```python
from build123d import *

# Parameters (mm, degrees)
SKETCH_1_W          = 20
SKETCH_1_H          = 20
SKETCH_1_R          = 1
EXTRUDE_1_DEPTH     = 28
EXTRUDE_2_DEPTH     = 1.6
SKETCH_3_R          = 2
EXTRUDE_3_DEPTH     = 18.4
CUT_EXTRUDE_1_DEPTH = 15


with BuildPart() as part:
    # 草图1 → 凸台-拉伸1 (new body)
    with BuildSketch(Plane(origin=(0, 0, 0), x_dir=(1, 0, 0), z_dir=(0, 1, 0))):
        with Locations((10, 10)):
            Rectangle(SKETCH_1_W, SKETCH_1_H)
        with Locations(Location((17.7, 2.3, 0), (0, 0, 270))):
            Circle(SKETCH_1_R, mode=Mode.SUBTRACT)
        with Locations(Location((17.7, 17.7, 0), (0, 0, 270))):
            Circle(SKETCH_1_R, mode=Mode.SUBTRACT)
        with Locations(Location((2.3, 17.7, 0), (0, 0, 270))):
            Circle(SKETCH_1_R, mode=Mode.SUBTRACT)
        with Locations(Location((2.3, 2.3, 0), (0, 0, 270))):
            Circle(SKETCH_1_R, mode=Mode.SUBTRACT)
    extrude(amount=EXTRUDE_1_DEPTH)

    # 草图2 → 凸台-拉伸2 (add)
    with BuildSketch(Plane(origin=(0, 28, 0), x_dir=(1, 0, 0), z_dir=(0, 1, 0))):
        with BuildLine():
            ThreePointArc((2, 10), (10, 2), (18, 10))
            Line((18, 10), (2, 10))
        make_face()
        with BuildLine():
            Line((2, 10), (18, 10))
            ThreePointArc((18, 10), (10, 18), (2, 10))
        make_face()
    extrude(amount=EXTRUDE_2_DEPTH)

    # 草图3 → 凸台-拉伸3 (add)
    with BuildSketch(Plane(origin=(0, 29.6, 0), x_dir=(1, 0, 0), z_dir=(0, 1, 0))):
        with Locations(Location((10, 10, 0), (0, 0, 270))):
            Circle(SKETCH_3_R)
    extrude(amount=EXTRUDE_3_DEPTH)

    # 草图4 → 切除-拉伸1 (cut)
    with BuildSketch(Plane(origin=(0, 48, 0), x_dir=(1, 0, 0), z_dir=(0, 1, 0))):
        with BuildLine():
            Line((11.481279617, 11.304155273), (11.481279617, 10))
            Line((11.481279617, 10), (11.481279617, 8.695844727))
            ThreePointArc((11.481279617, 8.695844727), (11.846406131, 9.303010274), (11.97357804, 10))
            ThreePointArc((11.97357804, 10), (11.846406131, 10.696989726), (11.481279617, 11.304155273))
        make_face()
    extrude(amount=-CUT_EXTRUDE_1_DEPTH, mode=Mode.SUBTRACT)


solid = part.part
```
Source: CAD feature listing. Evaluate the final solid. Frame: model axes, mm. A direction names the side the tool comes from. Give positions to 0.01 mm unless a question says otherwise; leave off trailing zeros. Write each loop counter-clockwise with the first axis right and the second up, starting at its lowest first coordinate (ties: lowest second). Pieces come first, ordered by that corner, then holes.
1. Section query B-B (x = 10). Return the cut outline in (y, z), then the cut area to 3 significant figures.
2. Section query D-D (y = 41). Return the cut outline in (x, z).
3. First-contact query: pin 1 (1.3 mm diameter, centred on y = 37.5, z = -10.5, fed in from +X); pin 2 (2.5 mm diameter, centred on x = 17.7, z = -2.3, fed in from +Y). Flat tips, straight axial feed; report the tip coordinate or a pass-through.
4. Pull-direction query (X, two-part tool) for faces 3 (the face through (20, 14, -10)), 4 (the face through (10, 14, 0)), 5 (the face through (1.917, 13.804, -16.776)); classes: +X half, -X half, draft (parallel to the pull), parting line (faces both ways), or undercut.
5. Section query C-C (z = -4.5). Return the cut outline in (x, y).
6. Access query for faces 1 (the face through (8.27, 28.79, -2.19)), 2 (the face through (10, 14, -20)). Directions: +Z, -Z, +X, -X, +Y, -Y. A direction counts if a zero-diameter tool reaches every point of the face in a straight line with its end or side. Return the directions, or none.
7. Section query A-A (y = 23). Return the cut outline in (x, z), then the cut area to 3 significant figures.
8. Material intervals for line 1 along X through (y, z) = (16.25, -17.7); line 2 along Y through (x, z) = (6.25, -5.5); line 3 along Y through (x, z) = (15.5, -1), sorted ascending.
Output values:
1. outline: (0, -20) - (28, -20) - (28, -18) - (29.6, -18) - (29.6, -12) - (48, -12) - (48, -8) - (29.6, -8) - (29.6, -2) - (28, -2) - (28, 0) - (0, 0) - close
1. area: 659 mm2
2. outline: circle Ø4 at (10, -10); hole (11.48, -11.3) arc R1.97 ccw to (11.48, -8.7) - close
3. pin 1: stops at x = 12
3. pin 2: stops at y = 28
4. face 3: +X half
4. face 4: draft
4. face 5: undercut
5. outline: (0, 0) - (20, 0) - (20, 28) - (15.81, 28) - (15.81, 29.6) - (4.19, 29.6) - (4.19, 28) - (0, 28) - close
6. face 1: +Y
6. face 2: -Z, +X, -X, +Y, -Y
7. outline: (0, -20) - (20, -20) - (20, 0) - (0, 0) - close; hole circle Ø2 at (2.3, -17.7); hole circle Ø2 at (2.3, -2.3); hole circle Ø2 at (17.7, -17.7); hole circle Ø2 at (17.7, -2.3)
7. area: 387 mm2
8. line 1: x = 0 to 1.3, 3.3 to 16.7, 18.7 to 20
8. line 2: y = 0 to 29.6
8. line 3: y = 0 to 28
